The model under review builds one solid part; all positions refer to its coordinate system, in mm. A direction names the side the tool comes from. Give positions to 0.01 mm unless a question says otherwise; leave off trailing zeros. Order: outer loops, then holes, each group sorted by start corner. A loop starts at its lowest first (then second) coordinate and runs counter-clockwise, first axis right, second up. Notation, with made-up numbers: (-37, 24) -> (11, 24) arc R22 cw to (11, 37) -> close; hole circle Ø5 at (71.25, 63). An arc over 180 degrees is marked (long way). Use one line per item in the form item = value.
```python
from build123d import *

# Parameters (mm, degrees)
SKETCH_1_R               = 19.8
EXTRUDE_1_DEPTH          = 13
SKETCH_2_R               = 19.8
EXTRUDE_2_DEPTH          = 3
SKETCH_3_W               = 60
SKETCH_3_H               = 24.618420452
EXTRUDE_3_DEPTH          = 3
FILLET_1_R               = 2
CUT_EXTRUDE_1_DEPTH      = 10
CUT_EXTRUDE_1_DEPTH_BACK = 10
SKETCH_4_R               = 1.821717012


with BuildPart() as part:
    # 草图1 → 凸台-拉伸1 (new body)
    with BuildSketch(Plane.XY):
        with Locations(Location((0, 0, 0), (0, 0, 180))):
            Circle(SKETCH_1_R)
        Polygon((0, -12.5), (12.5, -12.5), (12.5, 12.5), (0, 12.5), (-12.5, 12.5), (-12.5, -12.5), align=None, mode=Mode.SUBTRACT)
    extrude(amount=EXTRUDE_1_DEPTH)

    # 草图2 → 凸台-拉伸2 (add)
    # profile 1 of 5: a face of its own
    with BuildSketch(Plane(origin=(0, 0, 0), x_dir=(-1, 0, 0), z_dir=(0, 0, -1))):
        with BuildLine():
            ThreePointArc((30, 0), (0, 30), (-30, 0))
            Line((-30, 0), (-30, -41))
            Line((-30, -41), (30, -41))
            Line((30, -41), (30, 0))
        make_face()
        Circle(SKETCH_2_R, mode=Mode.SUBTRACT)
    # profile 2 of 5: a face of its own
    with BuildSketch(Plane(origin=(0, 0, 0), x_dir=(-1, 0, 0), z_dir=(0, 0, -1))):
        with BuildLine():
            Line((-12.5, 12.5), (-12.5, 11.5))
            ThreePointArc((-12.5, 11.5), (-12.207106781, 12.207106781), (-11.5, 12.5))
            Line((-11.5, 12.5), (-12.5, 12.5))
        make_face()
    # profile 3 of 5: a face of its own
    with BuildSketch(Plane(origin=(0, 0, 0), x_dir=(-1, 0, 0), z_dir=(0, 0, -1))):
        with BuildLine():
            ThreePointArc((12.5, -11.5), (12.207106781, -12.207106781), (11.5, -12.5))
            Line((11.5, -12.5), (12.5, -12.5))
            Line((12.5, -12.5), (12.5, -11.5))
        make_face()
    # profile 4 of 5: a face of its own
    with BuildSketch(Plane(origin=(0, 0, 0), x_dir=(-1, 0, 0), z_dir=(0, 0, -1))):
        with BuildLine():
            Line((-12.5, -12.5), (-11.5, -12.5))
            ThreePointArc((-11.5, -12.5), (-12.207106781, -12.207106781), (-12.5, -11.5))
            Line((-12.5, -11.5), (-12.5, -12.5))
        make_face()
    # profile 5 of 5: a face of its own
    with BuildSketch(Plane(origin=(0, 0, 0), x_dir=(-1, 0, 0), z_dir=(0, 0, -1))):
        with BuildLine():
            ThreePointArc((11.5, 12.5), (12.207106781, 12.207106781), (12.5, 11.5))
            Line((12.5, 11.5), (12.5, 12.5))
            Line((12.5, 12.5), (11.5, 12.5))
        make_face()
    extrude(amount=-EXTRUDE_2_DEPTH)

    # 草图3 → 凸台-拉伸3 (add)
    with BuildSketch(Plane(origin=(0, 0, 0), x_dir=(-1, 0, 0), z_dir=(0, 0, -1))):
        with Locations((0, -28.690789774)):
            Rectangle(SKETCH_3_W, SKETCH_3_H)
    extrude(amount=EXTRUDE_3_DEPTH)

    # 圆角1
    fillet_1_edges = [part.edges().sort_by_distance(p)[0] for p in [
        (30, -28.690789774, -3),
        (0, -41, -3),
        (-30, -28.690789774, -3),
        (0, -16.381579548, -3),
    ]]
    fillet(fillet_1_edges, radius=FILLET_1_R)

    # 草图4 → 切除-拉伸1 (cut, two sides: drawn at the far end of the back side and taken through both)
    with BuildSketch(Plane(origin=(0, 0, 0), x_dir=(-1, 0, 0), z_dir=(0, 0, -1)).offset(-CUT_EXTRUDE_1_DEPTH_BACK)):
        with Locations((20.33925745, -11.208047119)):
            Circle(SKETCH_4_R)
    extrude(amount=CUT_EXTRUDE_1_DEPTH + CUT_EXTRUDE_1_DEPTH_BACK, mode=Mode.SUBTRACT)


solid = part.part
```
1. Add section B-B on z = 9.75. Give the boundary of the cut face in (x, y), then the cut area to 3 significant figures.
Values:
outline = circle Ø39.6 at (0, 0); hole (-12.5, -12.5) -> (12.5, -12.5) -> (12.5, 12.5) -> (-12.5, 12.5) -> close
area = 607 mm^2
2. Add section D-D on y = 1.5. Give the boundary of the cut face in (x, z), then the cut area to 3 significant figures.
Values:
outline = (-29.96, 0) -> (-12.5, 0) -> (-12.5, 13) -> (-19.74, 13) -> (-19.74, 3) -> (-29.96, 3) -> close; (12.5, 0) -> (29.96, 0) -> (29.96, 3) -> (19.74, 3) -> (19.74, 13) -> (12.5, 13) -> close
area = 250 mm^2
3. The part is to be moulded in two halves that separate along Y. For faces 4 (the face through (-0.42, -16.952, -2.399)), 5 (the face through (-0.42, -40.43, -2.4)), 6 (the face through (-12.5, 0, 6)), say which applies: +Y half, -Y half, draft (parallel to the pull), parting line (faces both ways), or undercut.
Values:
face_4 = +Y half
face_5 = -Y half
face_6 = undercut
4. Add section C-C on y = -35. Give the boundary of the cut face in (x, z), then the cut area to 3 significant figures.
Values:
outline = (-30, -1) arc R2 ccw to (-28, -3) -> (28, -3) arc R2 ccw to (30, -1) -> (30, 3) -> (-30, 3) -> close
area = 358 mm^2
5. Tool access review of faces 1 (the face through (-18.9, -5.9, 7.9)), 2 (the face through (-30, -21, 1)), 3 (the face through (0, 17, 0)): name each direction out of +Z, -Z, +X, -X, +Y, -Y from which nothing blocks a thin tool from reaching the whole face with its end or side.
Values:
face_1 = +Z
face_2 = +Z, -Z, -X, +Y, -Y
face_3 = -Z, +X, -X, +Y
6. For pin 1 Ø1.1 at (x, y) = (-12, 12) entering from +Z; pin 2 Ø0.5 at (x, z) = (-5.5, -0.5) entering from +Y; pin 3 Ø8 at (x, z) = (-21.5, 8.5) entering from -Y; pin 4 Ø4 at (x, z) = (5.5, 8.5) entering from -Y, all flat-tipped, find the tip position at first contact; note any pin that passes through.
Values:
pin_1 = 13
pin_2 = -16.38
pin_3 = -9.26
pin_4 = -19.49
7. Add section A-A on x = 0. Give the boundary of the cut face in (y, z), then the cut area to 3 significant figures.
Values:
outline = (-41, -1) arc R2 ccw to (-39, -3) -> (-18.38, -3) arc R2 ccw to (-16.38, -1) -> (-16.38, 0) -> (-12.5, 0) -> (-12.5, 13) -> (-19.8, 13) -> (-19.8, 3) -> (-41, 3) -> close; (12.5, 0) -> (30, 0) -> (30, 3) -> (19.8, 3) -> (19.8, 13) -> (12.5, 13) -> close
area = 356 mm^2
8. For L1, parallel to X at y = -3.5, z = 1.5; L2, parallel to Z at x = -3.5, y = 24; L3, parallel to X at y = -11.5, z = 2.25, list the stretches that pass through material, from the lowest coordinate up.
Values:
L1 = -30 to -12.5, 12.5 to 30
L2 = 0 to 3
L3 = -30 to -22.14, -18.54 to -12.5, 12.5 to 30
